Model file for the job. Use its own axes, mm. Coordinates: 2 decimals unless noted, no trailing zeros. Loops run counter-clockwise (first coordinate to the right, second up) from the corner with the lowest first, then second, coordinate; pieces in that order, holes last.
from build123d import *

# Parameters (mm, degrees)
SKETCH_1_R               = 3
EXTRUDE_1_DEPTH          = 0.7
PATTERN_CIRCULAR_1_COUNT = 8
SKETCH_3_R               = 1
CUT_EXTRUDE_1_DEPTH      = 5.326950427


with BuildPart() as part:
    # 草图1 → 凸台-拉伸1 (new body)
    with BuildSketch(Plane.XY):
        Circle(SKETCH_1_R)
    extrude(amount=EXTRUDE_1_DEPTH)

    # 草图2 → 旋转1 (revolve)
    with BuildSketch(Plane.XY.offset(0.35)):
        with BuildLine():
            Line((0, 2.5), (0, 1.5))
            ThreePointArc((0, 1.5), (-0.5, 2), (0, 2.5))
        make_face()
    revolve_1 = revolve(axis=Axis((0, 2.5, 0.35), (0, -1, 0)))

    # 阵列(圆周)1: 旋转1 ×8 about axis
    pattern_circular_1_axis = Axis((0, -0.02874049, 0), (0, 0, 1))
    for i in range(1, PATTERN_CIRCULAR_1_COUNT):
        add(revolve_1.rotate(pattern_circular_1_axis, i * 360 / PATTERN_CIRCULAR_1_COUNT))

    # 草图3 → 切除-拉伸1 (cut, through all)
    with BuildSketch(Plane.XY.offset(0.7)):
        Circle(SKETCH_3_R)
    extrude(amount=-CUT_EXTRUDE_1_DEPTH, mode=Mode.SUBTRACT)


solid = part.part
Q1. Slice it at C-C (z = 0.6). List the corners of the cut face in (x, y), and give its area (3 significant figures).
Answers:
outline: circle Ø6 at (0, 0); hole circle Ø2 at (0, 0)
area: 25.1 mm2
Q2. Slice it at B-B (y = 0). List the corners of the cut face in (x, z), and give its area (3 significant figures).
Answers:
outline: (-3, 0) - (-2.38, 0) arc R0.5 ccw to (-1.67, 0) - (-1, 0) - (-1, 0.7) - (-1.67, 0.7) arc R0.5 ccw to (-2.38, 0.7) - (-3, 0.7) - close; (1, 0) - (1.67, 0) arc R0.5 ccw to (2.38, 0) - (3, 0) - (3, 0.7) - (2.38, 0.7) arc R0.5 ccw to (1.67, 0.7) - (1, 0.7) - close
area: 3.09 mm2
Q3. Flat gauge pin, fed straight in: P1, Ø2.5, axis at x = 0, y = 0, coming from the -Z side. Where does the tip first touch, or does it go through?
Answers:
P1: stops at z = 0
Q4. Slice it at D-D (x = -1.95). List the corners of the cut face in (y, z), and give its area (3 significant figures).
Answers:
outline: (-2.28, 0) - (-0.38, 0) arc R0.49 ccw to (0.32, 0) - (2.28, 0) - (2.28, 0.7) - (0.32, 0.7) arc R0.49 ccw to (-0.38, 0.7) - (-2.28, 0.7) - close
area: 3.33 mm2
Q5. Slice it at A-A (x = 0). List the corners of the cut face in (y, z).
Answers:
outline: (-3, 0) - (-2.41, 0) arc R0.5 ccw to (-1.7, 0) - (-1, 0) - (-1, 0.7) - (-1.7, 0.7) arc R0.5 ccw to (-2.41, 0.7) - (-3, 0.7) - close; (1, 0) - (1.64, 0) arc R0.5 ccw to (2.36, 0) - (3, 0) - (3, 0.7) - (2.36, 0.7) arc R0.5 ccw to (1.64, 0.7) - (1, 0.7) - close
Q6. Mould opens along Y. For faces 1 (the cylindrical face through (-0.217, -0.976, 0.355)), 2 (the flat face through (-1, 1, 0)), 3 (the cylindrical face through (-3, 0.1, 0.3)) say: +Y half, -Y half, draft (parallel to the pull), parting line (faces both ways), or undercut.
Answers:
face 1: undercut
face 2: undercut
face 3: parting line
Q7. Drill centre lines: line 1 (Y direction, x = 0, z = 0.2); line 2 (Z direction, x = 0.15, y = 1.2). Where is each one in solid material? Low to high.
Answers:
line 1: y = -3 to -1, 1 to 3
line 2: z = 0 to 0.7
